from build123d import *

# Parameters (mm, degrees)
BOSS_EXTRUDE1_DEPTH = 3
SKETCH2_R           = 5
SKETCH2_R_2         = 1
BOSS_EXTRUDE2_DEPTH = 3
CUT_EXTRUDE1_START  = -10
SKETCH7_R           = 1
CUT_EXTRUDE1_DEPTH  = 10
CUT_EXTRUDE2_START  = -10
SKETCH8_R           = 1
CUT_EXTRUDE2_DEPTH  = 10
SKETCH5_R           = 2.5
BOSS_EXTRUDE3_DEPTH = 3.41
SKETCH9_W           = 30.62
SKETCH9_H           = 3
BOSS_EXTRUDE4_DEPTH = 3.8
SKETCH10_W          = 30.62
SKETCH10_H          = 8
BOSS_EXTRUDE5_DEPTH = 3
FILLET3_R           = 2


with BuildPart() as part:
    # Sketch1 → Boss-Extrude1 (new body)
    with BuildSketch(Plane.XY):
        with BuildLine():
            Line((-64.206162528, 9.215011287), (85.023837472, 9.215011287))
            ThreePointArc((85.023837472, 9.215011287), (90.023837472, 4.215011287), (85.023837472, -0.784988713))
            Line((85.023837472, -0.784988713), (-64.206162528, -0.784988713))
            ThreePointArc((-64.206162528, -0.784988713), (-69.206162528, 4.215011287), (-64.206162528, 9.215011287))
        make_face()
    extrude(amount=BOSS_EXTRUDE1_DEPTH)

    # Sketch2 → Boss-Extrude2 (add)
    # profile 1 of 2: a face of its own
    with BuildSketch(Plane.XY.offset(3)):
        with Locations(Location((-64.206162528, 4.215011287, 0), (0, 0, 270))):
            Circle(SKETCH2_R)
        with Locations((-64.206162528, 4.215011287)):
            Circle(SKETCH2_R_2, mode=Mode.SUBTRACT)
    # profile 2 of 2: a face of its own
    with BuildSketch(Plane.XY.offset(3)):
        with Locations(Location((85.023837472, 4.215011287, 0), (0, 0, 90))):
            Circle(SKETCH2_R)
        with Locations((85.023837472, 4.215011287)):
            Circle(SKETCH2_R_2, mode=Mode.SUBTRACT)
    extrude(amount=BOSS_EXTRUDE2_DEPTH)

    # Sketch7 → Cut-Extrude1 (cut)
    with BuildSketch(Plane.XY.offset(6).offset(CUT_EXTRUDE1_START)):
        with Locations((-64.206162528, 4.215011287)):
            Circle(SKETCH7_R)
    extrude(amount=CUT_EXTRUDE1_DEPTH, mode=Mode.SUBTRACT)

    # Sketch8 → Cut-Extrude2 (cut)
    with BuildSketch(Plane.XY.offset(6).offset(CUT_EXTRUDE2_START)):
        with Locations((85.023837472, 4.215011287)):
            Circle(SKETCH8_R)
    extrude(amount=CUT_EXTRUDE2_DEPTH, mode=Mode.SUBTRACT)

    # Sketch5 → Boss-Extrude3 (add)
    with BuildSketch(Plane(origin=(0, 9.215011287, 0), x_dir=(1, 0, 0), z_dir=(0, 1, 0))):
        with BuildLine():
            Line((-4.901162528, -3), (25.718837472, -3))
            Line((25.718837472, -3), (25.718837472, -16.94))
            Line((25.718837472, -16.94), (25.718837472, -32.25))
            ThreePointArc((25.718837472, -32.25), (10.408837472, -47.56), (-4.901162528, -32.25))
            Line((-4.901162528, -32.25), (-4.901162528, -16.94))
            Line((-4.901162528, -16.94), (-4.901162528, -3))
        make_face()
        with Locations(Location((10.408837472, -32.25, 0), (0, 0, 270))):
            Circle(SKETCH5_R, mode=Mode.SUBTRACT)
    extrude(amount=-BOSS_EXTRUDE3_DEPTH)

    # Sketch9 → Boss-Extrude4 (add)
    with BuildSketch(Plane.XZ.offset(0.784988713)):
        with Locations((10.408837472, 1.5)):
            Rectangle(SKETCH9_W, SKETCH9_H)
    extrude(amount=BOSS_EXTRUDE4_DEPTH)

    # Sketch10 → Boss-Extrude5 (add)
    with BuildSketch(Plane.XZ.offset(4.584988713)):
        with Locations((10.408837472, 4)):
            Rectangle(SKETCH10_W, SKETCH10_H)
    extrude(amount=BOSS_EXTRUDE5_DEPTH)

    # Fillet3
    # the kernel refuses this fillet: 2 mm, written as the material it takes off along each edge
    with BuildSketch(Plane(origin=(25.718837472, 9.215011287, 3), x_dir=(-1, 0, 0), z_dir=(0, 0, 1)), Plane(origin=(-4.901162528, 9.215011287, 32.25), x_dir=(1, 0, 0), z_dir=(0, 0, -1))) as fillet3_piece_1:
        with BuildLine():
            CenterArc((FILLET3_R, FILLET3_R), FILLET3_R, 180, 90)
            Line((0, FILLET3_R), (0, 0))
            Line((0, 0), (FILLET3_R, 0))
        make_face()
    extrude(amount=29.25, mode=Mode.SUBTRACT)
    with BuildSketch(Plane(origin=(10.408837472, 9.215011287, 32.25), x_dir=(1, 0, 0), z_dir=(0, 0, -1))) as fillet3_piece_2:
        with BuildLine():
            CenterArc((15.31 - FILLET3_R, FILLET3_R), FILLET3_R, 270, 90)
            Line((15.31, FILLET3_R), (15.31, 0))
            Line((15.31, 0), (15.31 - FILLET3_R, 0))
        make_face()
    revolve(axis=Axis((10.408837472, 9.215011287, 32.25), (0, -1, 0)), revolution_arc=180, mode=Mode.SUBTRACT)
    with BuildSketch(Plane(origin=(-4.901162528, 0.415011287, 8), x_dir=(0, 0, -1), z_dir=(0, -1, 0)), Plane(origin=(25.718837472, 0.415011287, 8), x_dir=(-1, 0, 0), z_dir=(0, -1, 0))) as fillet3_piece_3:
        with BuildLine():
            CenterArc((FILLET3_R, FILLET3_R), FILLET3_R, 180, 90)
            Line((0, FILLET3_R), (0, 0))
            Line((0, 0), (FILLET3_R, 0))
        make_face()
    extrude(amount=13, mode=Mode.SUBTRACT)


solid = part.part
The listing builds one solid part. Answer for the finished solid, in the listing's coordinates (mm). A direction names the side the tool comes from. Coordinates: 2 decimals unless noted, no trailing zeros. Write each loop counter-clockwise with the first axis right and the second up, starting at its lowest first coordinate (ties: lowest second). Pieces come first, ordered by that corner, then holes. Notation, with made-up numbers: M 57.25,43.5 L 83.25,43.5 A28 ccw 83.25,82.5 Z; hole C 51.25,85.5 d1. An arc over 180 degrees is marked long. Put each result on its own line as item: value. Start each with the question number.
1. A cutting plane is placed at B-B on y = -2.75. Write down the section's boundary in (x, z).
2. A cutting plane is placed at C-C on x = 75. Write down the section's boundary in (y, z), then the cut area to 3 significant figures.
3. Flat-ended cylindrical pins translate along their axes: P1, Ø1.1, axis at y = 6.5, z = 18.5, coming from the +X side; P2, Ø0.9, axis at x = -30.5, z = 1.5, coming from the -Y side (3 decimals); P3, Ø0.7, axis at y = 6.5, z = 11, coming from the -X side. Find the tip coordinate at first contact, or state that the pin passes through.
4. Consider line 1 (X direction, y = 7.05, z = 32.25); line 2 (Y direction, x = 10, z = 7); line 3 (Z direction, x = 39, y = 2). Determine where each line is inside the solid, lowest interval first. Write a range as from..to.
5. Which of the six approach directions +Z, -Z, +X, -X, +Y, -Y give full straight-line access (tool end or side, diameter ignored) to faces 1 (the cylindrical face through (89.905, 3.131, 3.625)), 2 (the flat face through (-64, 3, 6)), 3 (the flat face through (-4.901, -5, 2))?
6. A cutting plane is placed at A-A on z = 10.5. Write down the section's boundary in (x, y), then the cut area to 3 significant figures.
7. For a pull along X with two mould halves and no side action, classify faces 4 (the cylindrical face through (8.888, 7.534, 30.266)), 5 (the flat face through (11, 4, 3)), 6 (the flat face through (25.719, -5, 2)), 7 (the flat face through (83.8, 4.1, 6)) as pulls with the +X half, pulls with the -X half, needs draft (parallel to the pull), parting line crosses it, or undercut.
Resolved:
1. outline: M -4.9,0 L 25.72,0 L 25.72,3 L -4.9,3 Z
2. outline: M -0.78,0 L 9.22,0 L 9.22,3 L -0.78,3 Z
2. area: 30.0 mm2
3. P1: stops at x = 25.72
3. P2: stops at y = -0.785
3. P3: stops at x = -4.9
4. line 1: x = -4.9..7.91, 12.91..25.72
4. line 2: y = -7.58..-4.58, 5.81..9.22
4. line 3: z = 0..3
5. face 1: +Z
5. face 2: +Z, -X, +Y, -Y
5. face 3: +Z, -Z, -X, -Y
6. outline: M -4.9,5.81 L 25.72,5.81 L 25.72,7.22 A2 ccw 23.72,9.22 L -2.9,9.22 A2 ccw -4.9,7.22 Z
6. area: 103 mm2
7. face 4: undercut
7. face 5: undercut
7. face 6: pulls with the +X half
7. face 7: needs draft
